from build123d import *

# Parameters (mm, degrees)
F2_R           = 3
F5_D           = 6.5
F5_DEPTH       = 10
F5_TIP         = 1.9527970118
F5_ON_F3_D     = 6.5
F5_ON_F3_DEPTH = 10
F5_ON_F3_TIP   = 1.9527970118


with BuildPart() as f1:
    # F0 (on Front) → F1 (revolve)
    with BuildSketch(Plane.XZ):
        Polygon((0, -15), (0, 15), (-11, 15), (-11, 11), (-15, 11), (-15, -11), (-11, -11), (-11, -15), align=None)
    revolve(axis=Axis((0, 0, 0), (0, 0, -1)))

    # F2
    f2_edges = [f1.edges().sort_by_distance(p)[0] for p in [
        (11, 0, 11),
        (11, 0, -11),
    ]]
    fillet(f2_edges, radius=F2_R)

    # F5
    with Locations(Plane(origin=(0, 0, -15), x_dir=(1, 0, 0), z_dir=(0, 0, -1))):
        with Locations((0, 0)):
            Hole(F5_D / 2, depth=F5_DEPTH)
            with Locations((0, 0, -(F5_DEPTH + F5_TIP / 2))):  # 118° drill point
                Cone(0, F5_D / 2, F5_TIP, mode=Mode.SUBTRACT)

    # F5 on F3
    with Locations(Plane.XY.offset(15)):
        with Locations((0, 0)):
            Hole(F5_ON_F3_D / 2, depth=F5_ON_F3_DEPTH)
            with Locations((0, 0, -(F5_ON_F3_DEPTH + F5_ON_F3_TIP / 2))):  # 118° drill point
                Cone(0, F5_ON_F3_D / 2, F5_ON_F3_TIP, mode=Mode.SUBTRACT)


solid = f1.part
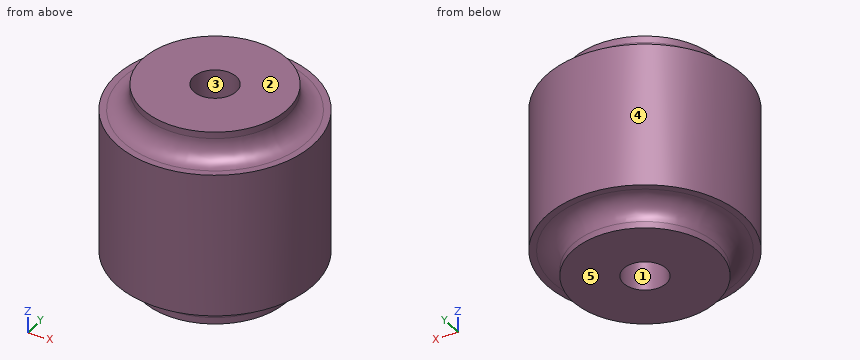
Here's how the part is built. I have some questions about the finished solid (model axes, mm). Face numbers are marked on the shaded views. A direction names the side the tool comes from. Coordinates: 2 decimals unless noted, no trailing zeros. Write each loop counter-clockwise with the first axis right and the second up, starting at its lowest first coordinate (ties: lowest second). Pieces come first, ordered by that corner, then holes.
Item 1: I want a section at A-A on z = 7.5. Write out the boundary of the cut face in (x, y), and give its area (3 significant figures).
Item 2: If I drill on line 1 (Y direction, x = 0, z = -10); line 2 (Y direction, x = 0, z = -11.75); line 3 (X direction, y = 2, z = -5.75), over which ranges is the centre line in solid material (lowest first)?
Item 3: I want a section at B-B on z = 1. Write out the boundary of the cut face in (x, y).
Item 4: Will these pins go through, and if not, where does the flat tip stop? pin 1 (1 mm diameter, centred on x = -3.5, z = 2, fed in from +Y); pin 2 (4 mm diameter, centred on x = 0, y = 0, fed in from -Z); pin 3 (4 mm diameter, centred on x = -8, z = 7.5, fed in from +Y).
Item 5: If we mould it in two halves opening along Y, with no side actions, what happens to the marked faces 3, 4 and 5? For each: +Y half, -Y half, draft (parallel to the pull), parting line (faces both ways), or undercut.
Item 6: On a 3-axis mill with a long thin cutter (end or side, diameter ignored), from which of +Z, -Z, +X, -X, +Y, -Y can I reach the whole of each face in a straight line? I mean the marked faces 1 and 2. Say none if no direction works.
Findings below:
1. outline: circle Ø30 at (0, 0); hole circle Ø6.5 at (0, 0)
1. area: 674 mm2
2. line 1: y = -15 to -3.25, 3.25 to 15
2. line 2: y = -12.02 to -3.25, 3.25 to 12.02
2. line 3: x = -14.87 to -2.56, 2.56 to 14.87
3. outline: circle Ø30 at (0, 0)
4. pin 1: stops at y = 14.7
4. pin 2: stops at z = -4.25
4. pin 3: stops at y = 13.75
5. face 3: undercut
5. face 4: parting line
5. face 5: draft
6. face 1: -Z
6. face 2: +Z, +X, -X, +Y, -Y
